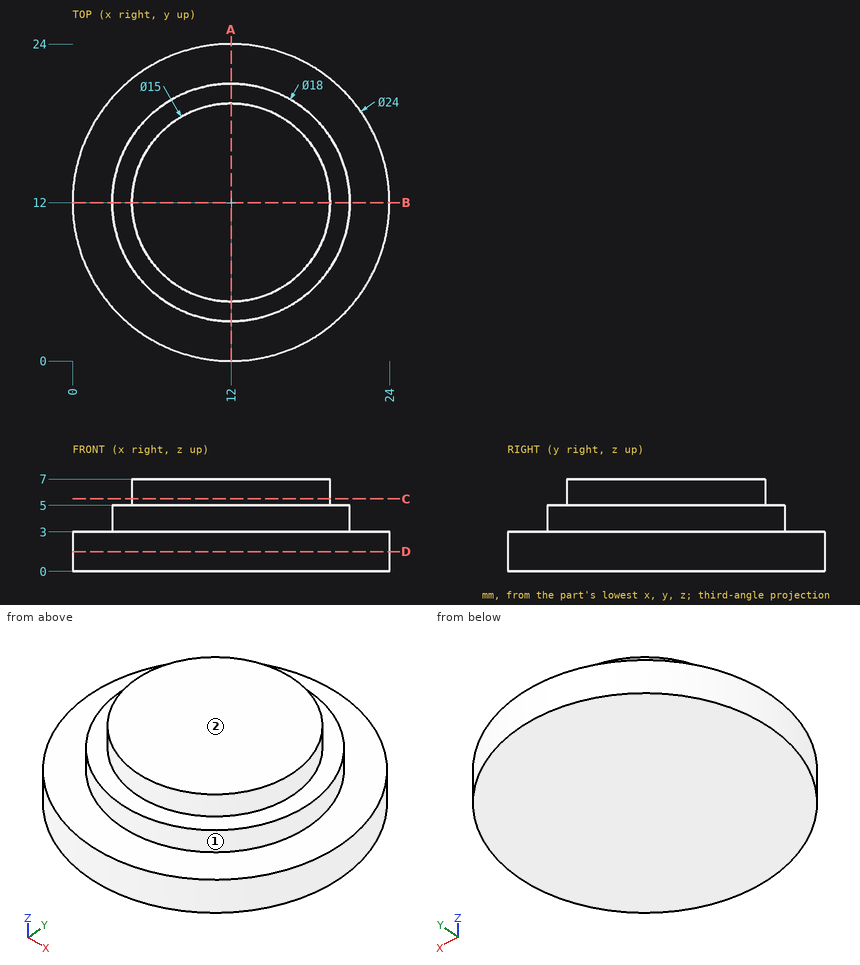
Geometry: see drawing. Coordinates: mm, zero at the bounding-box minimum. A direction names the side the tool comes from. Give positions to 0.01 mm unless a question says otherwise; leave off trailing zeros. Order: outer loops, then holes, each group sorted by start corner. A loop starts at its lowest first (then second) coordinate and runs counter-clockwise, first axis right, second up. Notation, with made-up numbers: (-39.5, 27.5) - (-22.5, 27.5) arc R14 cw to (-22.5, 33.5) - close; hole circle Ø7 at (-9.5, -36). An arc over 180 degrees is marked (long way). Use CSV: the item, a comma, the result in double quotes.
1. Section query D-D (z = 1.5). Output: boundary loops of the cut face in (x, y).
Answers below:
outline,"circle Ø24 at (12, 12)"
2. Access query for the marked faces 1 and 2. Directions: +Z, -Z, +X, -X, +Y, -Y. A direction counts if a zero-diameter tool reaches every point of the face in a straight line with its end or side. Return the directions, or none.
Answers below:
face 1,"+Z"
face 2,"+Z, +X, -X, +Y, -Y"
3. Section query A-A (x = 12). Output: boundary loops of the cut face in (y, z), plus the area to 3 significant figures.
Answers below:
outline,"(0, 0) - (24, 0) - (24, 3) - (21, 3) - (21, 5) - (19.5, 5) - (19.5, 7) - (4.5, 7) - (4.5, 5) - (3, 5) - (3, 3) - (0, 3) - close"
area,"138 mm2"
4. Section query C-C (z = 5.5). Output: boundary loops of the cut face in (x, y), plus the area to 3 significant figures.
Answers below:
outline,"circle Ø15 at (12, 12)"
area,"177 mm2"
5. Material intervals for line 1 along Z through (x, y) = (18.25, 2.5); line 2 along Z through (x, y) = (4.5, 13.5); line 3 along X through (y, z) = (11.75, 6), sorted ascending. Write a range as from..to.
Answers below:
line 1,"0..3"
line 2,"0..5"
line 3,"4.5..19.5"
6. Contact query for flat-ended pins moving along their axis: pin 1 (1 mm diameter, centred on x = 13.5, z = 2.5, fed in from -Y); pin 2 (3 mm diameter, centred on x = 20.5, z = 4, fed in from +Y); pin 3 (3 mm diameter, centred on y = 14, z = 3, fed in from -X). Output: stop coordinate, or through.
Answers below:
pin 1,"y = 0.04"
pin 2,"y = 21.46"
pin 3,"x = 0.01"
